from build123d import *

# Parameters (mm, degrees)
F0_W      = 88.9
F0_H      = 38.1
F1_DEPTH  = 42.8498
F3_DEPTH  = 127
F4_W      = 79.4004
F4_H      = 15.875
F5_DEPTH  = 6.35
F7_DEPTH  = 25.4
F9_DEPTH  = 127
F10_R     = 1.524
F12_DEPTH = 25.4
F13_R     = 1.27
F14_W     = 18.0139442934
F14_H     = 19.7421588048
F14_H_2   = 6.130434971
F15_DEPTH = 25.4


with BuildPart() as f1:
    # F0 (on Front) → F1 (new body)
    with BuildSketch(Plane.XZ):
        with Locations((44.45, 19.05)):
            Rectangle(F0_W, F0_H)
    extrude(amount=F1_DEPTH)

    # F2 (on face) → F3 (cut)
    with BuildSketch(Plane(origin=(0, 0, 0), x_dir=(0, -1, 0), z_dir=(-1, 0, 0))):
        Polygon((16.8691291251, 16.8691291251), (13.1255537659, 38.1), (0, 38.1), (0, 0), (5.515703716, 0), align=None)
        Polygon((16.3495332586, 38.1), (22.5383370557, 3.0015495405), (39.7230353842, 6.0316755111), (36.9663705637, 21.6654985902), (40.0931351795, 22.2168315543), (42.8498, 6.5830084752), (42.8498, 38.1), align=None)
    extrude(amount=-F3_DEPTH, mode=Mode.SUBTRACT)

    # F4 (on face) → F5 (cut)
    with BuildSketch(Plane(origin=(0, -42.6834811822, 7.526249363), x_dir=(1, 0, 0), z_dir=(0, -0.984807753, 0.1736481777))):
        with Locations((44.45, 6.9797081012)):
            Rectangle(F4_W, F4_H)
    extrude(amount=-F5_DEPTH, mode=Mode.SUBTRACT)

    # F6 (on face) → F7 (cut)
    with BuildSketch(Plane(origin=(0, -0.1663188178, -0.9432408877), x_dir=(1, 0, 0), z_dir=(0, 0.1736481777, 0.984807753))):
        Polygon((16.7943580049, -22.7171426803), (0, -22.7171426803), (0, -31.4420426803), align=None)
        Polygon((84.1502, -43.3419426803), (44.45, -22.7171426803), (4.7498, -43.3419426803), align=None)
        Polygon((88.9, -22.7171426803), (72.1056419951, -22.7171426803), (88.9, -31.4420426803), align=None)
    extrude(amount=-F7_DEPTH, mode=Mode.SUBTRACT)

    # F8 (on face) → F9 (cut)
    with BuildSketch(Plane(origin=(0, 0, 0), x_dir=(1, 0, 0), z_dir=(0, 0, -1))):
        Polygon((35.0774, 5.515703716), (16.7943580049, 23.0675912236), (0, 23.0675912236), (0, 5.515703716), align=None)
        Polygon((72.1056419951, 23.0675912236), (53.8226, 5.515703716), (88.9, 5.515703716), (88.9, 23.0675912236), align=None)
    extrude(amount=-F9_DEPTH, mode=Mode.SUBTRACT)

    # F10
    f10_edges = [f1.edges().sort_by_distance(p)[0] for p in [
        (44.45, -13.125554, 38.1),
        (44.45, -16.349533, 38.1),
        (2.3749, -36.966371, 21.665499),
        (2.3749, -40.093135, 22.216832),
        (86.5251, -36.966371, 21.665499),
        (86.5251, -40.093135, 22.216832),
    ]]
    fillet(f10_edges, radius=F10_R)

    # F11 (on face) → F12 (cut)
    with BuildSketch(Plane(origin=(0, 0, 0), x_dir=(1, 0, 0), z_dir=(0, 0, -1))):
        Polygon((16.7943580049, 23.0675912236), (0, 31.9270868696), (0, 30.7840723544), (16.1012234683, 21.7536620769), align=None)
        Polygon((88.9, 31.9270868696), (72.1056419951, 23.0675912236), (72.6024817226, 22.125765121), (88.9, 30.4145570844), align=None)
    extrude(amount=-F12_DEPTH, mode=Mode.SUBTRACT)

    # F13
    f13_edges = [f1.edges().sort_by_distance(p)[0] for p in [
        (44.45, -5.515704, 0),
        (85.42491, -42.8498, 0),
        (3.47509, -42.8498, 0),
    ]]
    fillet(f13_edges, radius=F13_R)

    # F14 (on face) → F15 (cut)
    with BuildSketch(Plane(origin=(0, -19.245253622, 3.3934574641), x_dir=(-1, 0, 0), z_dir=(0, 0.984807753, -0.1736481777))):
        with Locations((-44.45, 23.5546350199)):
            Rectangle(F14_W, F14_H)
        with Locations((-44.45, 36.4909319078)):
            Rectangle(F14_W, F14_H_2)
    extrude(amount=-F15_DEPTH, mode=Mode.SUBTRACT)


solid = f1.part
Can you work these out from the model? Positions are in its coordinate system, mm. A direction names the side the tool comes from. Round coordinates to 2 decimals unless told otherwise and drop trailing zeros. Write each loop counter-clockwise with the first axis right and the second up, starting at its lowest first coordinate (ties: lowest second). Pieces come first, ordered by that corner, then holes. Notation, with made-up numbers: (82.25, -8.5) - (139.25, -8.5) arc R19 ccw to (139.25, 15.5) - close; hole circle Ø4 at (-33, 78.5). An arc over 180 degrees is marked (long way). Write each question's results on one line, items separated by ' | '. Start each with the question number.
1) We'd pull the mould along X, two halves only. Please class faces 4 (the flat face through (20.467, -35.225, 2.803)), 5 (the flat face through (86, -42.85, 4)), 6 (the flat face through (35.443, -17, 27)), 7 (the flat face through (0, -40, 8)): released by +X, released by -X, zero draft, split by the parting line, or undercut.
2) Please list where these lines run through material, in increasing order: line 1 (X direction, y = -40.5, z = 19); line 2 (X direction, y = -17.5, z = 26); line 3 (Z direction, x = 53, y = -8).
3) Suppose I cut it at B-B (y = -28). List the corners of the cut face in (x, z) for me, and give its area (3 significant figures).
4) Suppose I cut it at C-C (z = 28). List the corners of the cut face in (x, y) for me.
5) Suppose I cut it at D-D (x = 41.5). List the corners of the cut face in (y, z) for me.
6) Suppose I cut it at A-A (z = 8). List the corners of the cut face in (x, y) for me, and give its area (3 significant figures).
7) For pin 1 Ø3 at (y, z) = (-19, 17.5) entering from -X; pin 2 Ø1.5 at (x, z) = (31.5, 22) entering from -Y; pin 3 Ø3.5 at (y, z) = (-16.5, 29.5) entering from +X, each with a flat end and sliding along its axis, tell me the tip position at first contact or that it passes through.
8) Which directions (+Z, -Z, +X, -X, +Y, -Y) give clear straight access to the entire face, cutting with the end or side of a thin tool? Please do faces 1 (the flat face through (44.58, -18.41, 17.14)), 2 (the flat face through (64.578, -33.253, 2.455)), 3 (the flat face through (30.62, -15.18, 26.45)).
Here are the results:
1) face 4: undercut | face 5: zero draft | face 6: undercut | face 7: released by -X
2) line 1: x = 0 to 4.75, 84.15 to 88.9 | line 2: x = 22.59 to 35.44, 53.46 to 66.31 | line 3: z = 0 to 3.69
3) outline: (7.44, 0) - (35.1, 0) - (33.77, 3.96) - (7.44, 3.96) - close; (53.8, 0) - (81.46, 0) - (81.46, 3.96) - (55.13, 3.96) - close | area: 214 mm2
4) outline: (21.94, -18.13) - (35.44, -18.13) - (35.44, -14.91) - (25.3, -14.91) - close; (53.46, -18.13) - (66.96, -18.13) - (63.6, -14.91) - (53.46, -14.91) - close
5) outline: (-24.62, 0) - (-7.9, 0) arc R1.27 ccw to (-6.85, 1.98) - (-16.87, 16.87) - (-20, 17.42) - (-22.54, 3) - (-24.05, 3.27) - close
6) outline: (0, -42.6) - (4.75, -42.6) - (4.75, -39.38) - (0, -39.38) - close; (18.26, -21.66) - (70.64, -21.66) - (59.43, -10.9) - (29.47, -10.9) - close; (84.15, -42.6) - (88.9, -42.6) - (88.9, -39.38) - (84.15, -39.38) - close | area: 473 mm2
7) pin 1: stops at x = 19.83 | pin 2: stops at y = -19.32 | pin 3: stops at x = 66.85
8) face 1: +Z, +Y | face 2: +Z, -Y | face 3: +X, -X, +Y
